Check sheet for the modelled part. Datum: model origin and axes. Units: mm. Face numbers are marked on the shaded views. A direction names the side the tool comes from. Coordinates: 2 decimals unless noted, no trailing zeros. Loops run counter-clockwise (first coordinate to the right, second up) from the corner with the lowest first, then second, coordinate; pieces in that order, holes last. Notation, with made-up numbers: M 34.5,68 L 74.5,68 A8 ccw 74.5,83 Z; hole C 62.25,58.25 d4. An arc over 180 degrees is marked long. Answer as CSV lines item,"result". Start each with the question number.
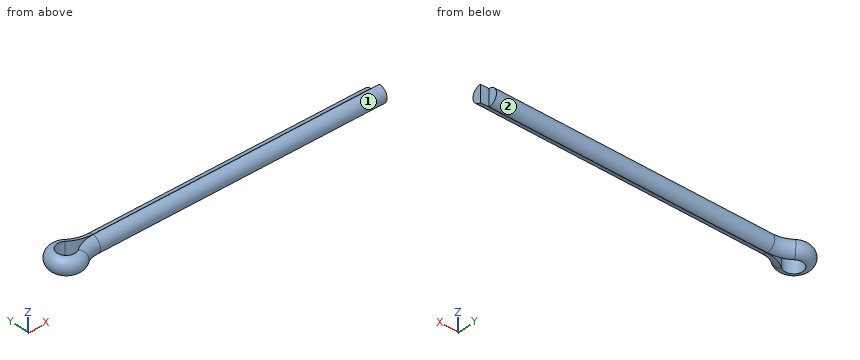
from build123d import *


with BuildPart() as part:
    # Sweep1: sweep along a path in Sketch3
    with BuildLine(Plane.XY) as sweep1_path:
        Line((0, 0.0254), (-50.8, 0.0254))
        ThreePointArc((-50.8, 0.0254), (-52.823920445, 0.356575694), (-54.636731203, 1.31555873))
        ThreePointArc((-54.636731203, 1.31555873), (-57.285281316, 0), (-54.636731203, -1.31555873))
        ThreePointArc((-54.636731203, -1.31555873), (-52.823920445, -0.356575694), (-50.8, -0.0254))
        Line((-50.8, -0.0254), (1.524, -0.0254))
    # Sketch4 → Sweep1 (sweep)
    with BuildSketch(Plane(origin=(0, 0, 0), x_dir=(0, 0, -1), z_dir=(1, 0, 0))):
        with BuildLine():
            Line((-1.523788319, 0.0254), (1.523788319, 0.0254))
            ThreePointArc((1.523788319, 0.0254), (0, 1.524), (-1.523788319, 0.0254))
        make_face()
    sweep(path=sweep1_path.line)


solid = part.part
Item 1: Sectioned sample at A-A, the plane z = 0.85. Record the boundary of the cut face in (x, y), and give its area (3 significant figures).
Item 2: Set-up check for the marked faces 1 and 2: record each of +Z, -Z, +X, -X, +Y, -Y from which the full face is reachable in a straight line by a thin tool's end or side.
Item 3: Material ranges on line 1 (Z direction, x = -22, y = 0.75); line 2 (Y direction, x = -53.5, z = -1.25); line 3 (X direction, y = 2, z = 0.7), recorded low to high. Write a range as from..to.
Item 4: Sectioned sample at B-B, the plane x = -28. Record the boundary of the cut face in (y, z).
Item 5: Go/stop test with flat-tipped pins: pin 1 (1.5 mm diameter, centred on x = -37, z = -0.5, fed in from +Y); pin 2 (0.7 mm diameter, centred on y = 1, z = 0, fed in from +X); pin 3 (2.5 mm diameter, centred on x = -55.63, y = 0, fed in from +Z); pin 4 (1 mm diameter, centred on y = 2, z = 1, fed in from -X). Record where each tip stops, or that it passes through.
Reply:
1,outline,"M -54.64,-1.32 A1.65 cw long -54.64,1.32 A6.35 ccw -50.8,0.03 L 0,0.03 L 0,1.26 L -50.8,1.26 A5.11 cw -53.89,2.3 A2.89 ccw long -53.89,-2.3 A5.11 cw -50.8,-1.26 L 1.52,-1.26 L 1.52,-0.03 L -50.8,-0.03 A6.35 ccw Z"
1,area,"150 mm²"
2,face 1,"+X, -Y"
2,face 2,"+X, +Y"
3,line 1,"-1.33..1.33"
3,line 2,"-1.58..-0.63, 0.63..1.58"
3,line 3,"-57.84..-53.26"
4,outline,"M -0.03,-1.52 L -0.03,1.52 A1.52 ccw Z; M 0.03,-1.52 A1.52 ccw 0.03,1.52 Z"
5,pin 1,"y = 1.52"
5,pin 2,"x = 0"
5,pin 3,"through"
5,pin 4,"x = -58.15"
